Could you check a few things on this model? Use its own coordinates, in mm. Round coordinates to 2 decimals unless told otherwise and drop trailing zeros. Loops run counter-clockwise (first coordinate to the right, second up) from the corner with the lowest first, then second, coordinate; pieces in that order, holes last.
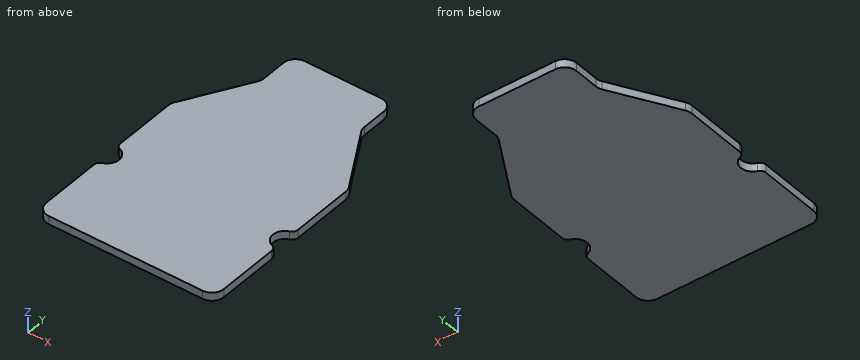
from build123d import *

# Parameters (mm, degrees)
BOSS_EXTRUDE1_DEPTH = 6.88
FILLET1_R           = 10
SKETCH2_R           = 10
CUT_EXTRUDE1_DEPTH  = 179.640923083
FILLET2_R           = 5


with BuildPart() as part:
    # Sketch1 → Boss-Extrude1 (new body)
    with BuildSketch(Plane.XY):
        Polygon((-74.65, 72.15), (-42.15, 128.441651246), (-42.15, 162.15), (-22.688475773, 162.15), (22.688475773, 162.15), (42.15, 162.15), (42.15, 128.441651246), (74.65, 72.15), (74.65, -72.15), (-74.65, -72.15), align=None)
    extrude(amount=BOSS_EXTRUDE1_DEPTH)

    # Fillet1
    fillet1_edges = [part.edges().sort_by_distance(p)[0] for p in [
        (-74.65, 72.15, 3.44),
        (-42.15, 128.441651246, 3.44),
        (-42.15, 162.15, 3.44),
        (42.15, 162.15, 3.44),
        (42.15, 128.441651246, 3.44),
        (74.65, 72.15, 3.44),
        (74.65, -72.15, 3.44),
        (-74.65, -72.15, 3.44),
    ]]
    fillet(fillet1_edges, radius=FILLET1_R)

    # Sketch2 → Cut-Extrude1 (cut, through all)
    with BuildSketch(Plane.XY.offset(6.88)):
        with Locations((-74.65, 3.660254038)):
            Circle(SKETCH2_R)
        with Locations((74.65, 3.660254038)):
            Circle(SKETCH2_R)
    extrude(amount=-CUT_EXTRUDE1_DEPTH, mode=Mode.SUBTRACT)

    # Fillet2
    fillet2_edges = [part.edges().sort_by_distance(p)[0] for p in [
        (-74.65, 13.660254038, 3.44),
        (-74.65, -6.339745962, 3.44),
        (74.65, -6.339745962, 3.44),
        (74.65, 13.660254038, 3.44),
    ]]
    fillet(fillet2_edges, radius=FILLET2_R)


solid = part.part
Item 1: If we section it at C-C, the plane y = 116.5: Please give me the cut outline in (x, z), then the cut area to 3 significant figures.
Results list:
outline: (-49.04, 0) - (49.04, 0) - (49.04, 6.88) - (-49.04, 6.88) - close
area: 675 mm2
Item 2: If we section it at B-B, the plane y = 147.5: Please give me the cut outline in (x, z), then the cut area to 3 significant figures.
Results list:
outline: (-42.15, 0) - (42.15, 0) - (42.15, 6.88) - (-42.15, 6.88) - close
area: 580 mm2
Item 3: If I drill on line 1 along Y through (x, z) = (43.5, 2.5); line 2 along X through (y, z) = (135, 4.5); line 3 along Y through (x, z) = (67, 4), over which ranges is the centre line in solid material (lowest first)?
Results list:
line 1: y = -72.15 to 126.1
line 2: x = -42.15 to 42.15
line 3: y = -71.87 to -2.78, 10.1 to 85.4
Item 4: If we section it at A-A, the plane z = 4: Please give me the cut outline in (x, y).
Results list:
outline: (-74.65, -62.15) arc R10 ccw to (-64.65, -72.15) - (64.65, -72.15) arc R10 ccw to (74.65, -62.15) - (74.65, -10.48) arc R5 ccw to (71.32, -5.77) arc R10 cw to (71.32, 13.09) arc R5 ccw to (74.65, 17.8) - (74.65, 69.47) arc R10 ccw to (73.31, 74.47) - (43.49, 126.12) arc R10 cw to (42.15, 131.12) - (42.15, 152.15) arc R10 ccw to (32.15, 162.15) - (-32.15, 162.15) arc R10 ccw to (-42.15, 152.15) - (-42.15, 131.12) arc R10 cw to (-43.49, 126.12) - (-73.31, 74.47) arc R10 ccw to (-74.65, 69.47) - (-74.65, 17.8) arc R5 ccw to (-71.32, 13.09) arc R10 cw to (-71.32, -5.77) arc R5 ccw to (-74.65, -10.48) - close
Item 5: Will this pin go through, and if not, where does the flat tip stop? pin 1 (3.5 mm diameter, centred on y = 140.5, z = 3.5, fed in from -X).
Results list:
pin 1: stops at x = -42.15
